Source: CAD feature listing. Evaluate the final solid. Frame: model axes, mm. Face numbers are marked on the shaded views. Round coordinates to 2 decimals unless told otherwise and drop trailing zeros. Loops run counter-clockwise (first coordinate to the right, second up) from the corner with the lowest first, then second, coordinate; pieces in that order, holes last. Notation, with made-up numbers: (83.25, 18) - (119.25, 18) arc R26 ccw to (119.25, 35) - close; hole circle Ø8 at (-18, -8). An arc over 180 degrees is marked (long way). One line per question, with ' | ' between items.
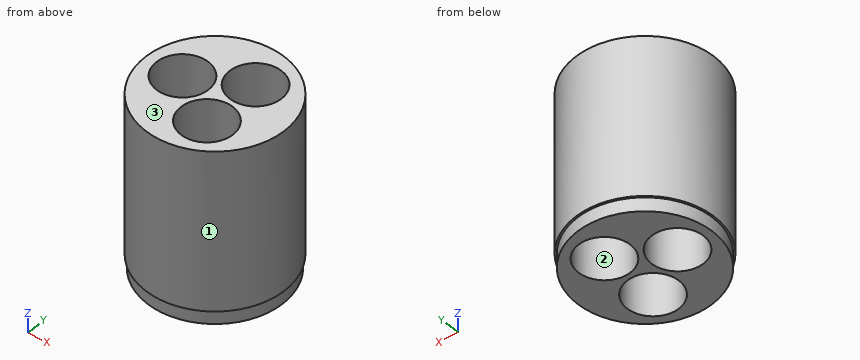
from build123d import *

# Parameters (mm, degrees)
F0_R     = 20
F1_DEPTH = 50
F2_R     = 7.5
F3_DEPTH = 50.001
F4_R     = 20
F4_R_2   = 19.5
F5_DEPTH = 4


with BuildPart() as f1:
    # F0 (on Top) → F1 (new body)
    with BuildSketch(Plane.XY):
        Circle(F0_R)
    extrude(amount=F1_DEPTH)

    # F2 (on face) → F3 (cut, through all)
    with BuildSketch(Plane(origin=(0, 0, 0), x_dir=(1, 0, 0), z_dir=(0, 0, -1))):
        with Locations((-9.5, 0)):
            Circle(F2_R)
        with Locations((4.75, -8.227241)):
            Circle(F2_R)
        with Locations((4.75, 8.227241)):
            Circle(F2_R)
    extrude(amount=-F3_DEPTH, mode=Mode.SUBTRACT)

    # F4 (on face) → F5 (cut)
    with BuildSketch(Plane(origin=(0, 0, 0), x_dir=(1, 0, 0), z_dir=(0, 0, -1))):
        Circle(F4_R)
        Circle(F4_R_2, mode=Mode.SUBTRACT)
    extrude(amount=-F5_DEPTH, mode=Mode.SUBTRACT)


solid = f1.part
1. Section query A-A, the plane x = -9.5. Return loops of the section in (y, z), plus the area to 3 significant figures.
Worked out:
outline: (-17.6, 4) - (-17.03, 4) - (-17.03, 0) - (-7.5, 0) - (-7.5, 50) - (-17.6, 50) - close; (7.5, 0) - (17.03, 0) - (17.03, 4) - (17.6, 4) - (17.6, 50) - (7.5, 50) - close | area: 1,010 mm2
2. Section query C-C, the plane x = 4.75. Return loops of the section in (y, z), plus the area to 3 significant figures.
Worked out:
outline: (-19.43, 4) - (-18.91, 4) - (-18.91, 0) - (-15.73, 0) - (-15.73, 50) - (-19.43, 50) - close; (-0.73, 0) - (0.73, 0) - (0.73, 50) - (-0.73, 50) - close; (15.73, 0) - (18.91, 0) - (18.91, 4) - (19.43, 4) - (19.43, 50) - (15.73, 50) - close | area: 439 mm2
3. Mould query, pull axis Y, two halves, no side actions, for the marked faces 1, 2 and 3. Classes: released by +Y, released by -Y, zero draft, split by the parting line, or undercut.
Worked out:
face 1: split by the parting line | face 2: undercut | face 3: zero draft
4. Section query D-D, the plane y = 5.5. Return loops of the section in (x, z), plus the area to 3 significant figures.
Worked out:
outline: (-19.23, 4) - (-18.71, 4) - (-18.71, 0) - (-14.6, 0) - (-14.6, 50) - (-19.23, 50) - close; (-4.4, 0) - (-2.24, 0) - (-2.24, 50) - (-4.4, 50) - close; (11.74, 0) - (18.71, 0) - (18.71, 4) - (19.23, 4) - (19.23, 50) - (11.74, 50) - close | area: 710 mm2
5. Section query B-B, the plane y = 13. Return loops of the section in (x, z), plus the area to 3 significant figures.
Worked out:
outline: (-15.2, 4) - (-14.53, 4) - (-14.53, 0) - (-1.04, 0) - (-1.04, 50) - (-15.2, 50) - close; (10.54, 0) - (14.53, 0) - (14.53, 4) - (15.2, 4) - (15.2, 50) - (10.54, 50) - close | area: 936 mm2
6. Contact query for flat-ended pins moving along their axis: P1, Ø5, axis at y = -10.5, z = 23, coming from the +X side; P2, Ø1, axis at x = -15.5, y = 0, coming from the -Z side; P3, Ø5, axis at x = -13.5, z = 18.5, coming from the +Y side; P4, Ø8, axis at y = -12.5, z = 16.5, coming from the +X side. Output: stop coordinate, or through.
Worked out:
P1: stops at x = 18.33 | P2: passes through | P3: stops at y = 16.7 | P4: stops at x = 18.1
7. Material intervals for probe 1 along X at (y, z) = (3.5, 35.5); probe 2 along Y at (x, z) = (10.5, 27); probe 3 along X at (y, z) = (0, 29), sorted ascending.
Worked out:
probe 1: x = -19.69 to -16.13, -2.87 to -1.07, 10.57 to 19.69 | probe 2: y = -17.02 to -13.04, -3.41 to 3.41, 13.04 to 17.02 | probe 3: x = -20 to -17, -2 to 20
